from build123d import *

# Parameters (mm, degrees)
F0_W     = 30
F0_H     = 30
F0_W_2   = 26
F0_H_2   = 26
F1_DEPTH = 60
F3_DEPTH = 3
F0_W_3   = 22.6
F0_H_3   = 22.6
F4_DEPTH = 2


with BuildPart() as f1:
    # F0 (on Top) → F1 (new body)
    with BuildSketch(Plane.XY):
        Rectangle(F0_W, F0_H)
        Rectangle(F0_W_2, F0_H_2, mode=Mode.SUBTRACT)
    extrude(amount=F1_DEPTH)

    # F2 (on face) → F3 (cut)
    with BuildSketch(Plane(origin=(0, 0, 0), x_dir=(1, 0, 0), z_dir=(0, 0, -1))):
        with BuildLine():
            ThreePointArc((-2.5, 0), (0, -2.5), (2.5, 0))
            ThreePointArc((2.5, 0), (0, 2.5), (-2.5, 0))
        make_face()
    extrude(amount=-F3_DEPTH, mode=Mode.SUBTRACT)

    # F0 (on Top) → F4 (join)
    with BuildSketch(Plane.XY):
        Rectangle(F0_W_2, F0_H_2)
        Rectangle(F0_W_3, F0_H_3, mode=Mode.SUBTRACT)
    extrude(amount=F4_DEPTH)


solid = f1.part
The listing builds one solid part. Answer for the finished solid, in the listing's coordinates (mm). A direction names the side the tool comes from. Coordinates: 2 decimals unless noted, no trailing zeros. Order: outer loops, then holes, each group sorted by start corner. A loop starts at its lowest first (then second) coordinate and runs counter-clockwise, first axis right, second up. Notation, with made-up numbers: (1, 66) -> (29, 66) arc R23 ccw to (29, 77) -> close; hole circle Ø5 at (37, 49). An arc over 180 degrees is marked (long way). Answer in a Markdown table with one row per item. Add a question column.
Item 1: Find section A-A (x = -8.75). Write down the section's boundary in (y, z).
Item 2: Which of the six approach directions +Z, -Z, +X, -X, +Y, -Y give full straight-line access (tool end or side, diameter ignored) to faces 1 (the face through (0, 13, 31)), 2 (the face through (-14, 0, 0)), 3 (the face through (-11.3, 0, 1))?
Item 3: Find the intervals of material crossed by L1, parallel to Y at x = -4.75, z = 47.5; L2, parallel to Z at x = 4, y = -11.5, in increasing order. Write a range as from..to.
Item 4: Determine the mould class of faces 4 (the face through (-15, 0, 30)), 5 (the face through (15, 0, 30)), 6 (the face through (-13, 0, 31)), 7 (the face through (0, -15, 30)) for opening direction X: +X half, -X half, draft (parallel to the pull), parting line (faces both ways), or undercut.
Item 5: Find section C-C (z = 35.5). Write down the section's boundary in (x, y).
Item 6: Each of these flat-tipped pins is pushed along its axis until it touches: P1, Ø12, axis at x = 11, y = -10, coming from the +Z side; P2, Ø13, axis at x = 0, y = -5, coming from the +Z side. Where does it stop, or does it pass through?
Result set:
| question | item | result |
|---|---|---|
| 1 | outline | (-15, 0) -> (-11.3, 0) -> (-11.3, 2) -> (-13, 2) -> (-13, 60) -> (-15, 60) -> close; (11.3, 0) -> (15, 0) -> (15, 60) -> (13, 60) -> (13, 2) -> (11.3, 2) -> close |
| 2 | face 1 | +Z |
| 2 | face 2 | -Z, +X, -X, +Y, -Y |
| 2 | face 3 | +Z, -Z |
| 3 | L1 | y = -15..-13, 13..15 |
| 3 | L2 | z = 0..2 |
| 4 | face 4 | -X half |
| 4 | face 5 | +X half |
| 4 | face 6 | undercut |
| 4 | face 7 | draft |
| 5 | outline | (-15, -15) -> (15, -15) -> (15, 15) -> (-15, 15) -> close; hole (-13, -13) -> (13, -13) -> (13, 13) -> (-13, 13) -> close |
| 6 | P1 | stops at z = 60 |
| 6 | P2 | stops at z = 2 |
